For this review, take the finished solid that the model builds, in its own axes (mm). A direction names the side the tool comes from. Round coordinates to 2 decimals unless told otherwise and drop trailing zeros. Write each loop counter-clockwise with the first axis right and the second up, starting at its lowest first coordinate (ties: lowest second). Pieces come first, ordered by that corner, then holes. Notation, with made-up numbers: (0.25, 13.25) - (22.25, 13.25) arc R19 ccw to (22.25, 22.25) - close; hole circle Ø1 at (-1, 82). An arc over 180 degrees is marked (long way). One line per item, written item: value. Start each with the question number.
Q1. Add section D-D on y = 15.5. Write out the cut boundary in (x, z), and give its area (3 significant figures).
Q2. Mouldability with a two-part tool opening along X and no side actions: class faces 4 (the face through (22.805, 25.487, 0.74)), 5 (the face through (38, 24, 1)), 6 (the face through (0, -14, 1)), 7 (the face through (19, 32.5, 1)) as +X half, -X half, draft (parallel to the pull), parting line (faces both ways), or undercut.
Q3. Add section A-A on x = 33. Write out the cut boundary in (y, z).
Q4. Tool access review of faces 1 (the face through (18, 0, 1)), 2 (the face through (2.6, 20.92, 0.76)), 3 (the face through (1.141, 31.297, 0.76)): name each direction out of +Z, -Z, +X, -X, +Y, -Y from which nothing blocks a thin tool from reaching the whole face with its end or side.
Q5. Add section B-B on z = 0.5. Write out the cut boundary in (x, y).
Q6. Add section C-C on y = 24. Write out the cut boundary in (x, z).
Q7. For probe 1 along Y at (x, z) = (33, 0.5); probe 2 along Y at (x, z) = (22, 0.9); probe 3 along X at (y, z) = (-25, 0.5), list the stretches that pass through material, from the lowest coordinate up.
```python
from build123d import *

# Parameters (mm, degrees)
ESQUISSE1_R             = 2.5
ESQUISSE1_R_2           = 1.5
BOSS_EXTRU_1_DEPTH      = 1.5
CONG_1_R                = 4
ENL_V_MAT_EXTRU_1_DEPTH = 51.024993753


with BuildPart() as part:
    # Esquisse1 → Boss.-Extru.1 (new body)
    with BuildSketch(Plane.XY):
        Polygon((38, -20), (38, -32.5), (0, -32.5), (0, 32.5), (38, 32.5), (38, 20), (18, 20), (18, -20), align=None)
        with Locations((8, 25)):
            Circle(ESQUISSE1_R, mode=Mode.SUBTRACT)
        with Locations((23, 24)):
            Circle(ESQUISSE1_R_2, mode=Mode.SUBTRACT)
        with Locations(Location((33, 24, 0), (0, 0, 180))):
            Circle(ESQUISSE1_R_2, mode=Mode.SUBTRACT)
        with Locations((33, -24)):
            Circle(ESQUISSE1_R_2, mode=Mode.SUBTRACT)
        with Locations(Location((23, -24, 0), (0, 0, 180))):
            Circle(ESQUISSE1_R_2, mode=Mode.SUBTRACT)
        with Locations(Location((8, -25, 0), (0, 0, 180))):
            Circle(ESQUISSE1_R, mode=Mode.SUBTRACT)
    extrude(amount=BOSS_EXTRU_1_DEPTH)

    # Congé1
    cong_1_edges = [part.edges().sort_by_distance(p)[0] for p in [
        (38, -32.5, 0.75),
        (0, -32.5, 0.75),
        (0, 32.5, 0.75),
        (38, 32.5, 0.75),
    ]]
    fillet(cong_1_edges, radius=CONG_1_R)

    # Esquisse2 → Enlèv. mat.-Extru.1 (cut, through all)
    with BuildSketch(Plane.XY.offset(1.5)):
        Polygon((0, 21.617026009), (5.268332191, 20.205380653), (0, 0.543697246), align=None)
    extrude(amount=-ENL_V_MAT_EXTRU_1_DEPTH, mode=Mode.SUBTRACT)


solid = part.part
```
Result set:
1. outline: (4.01, 0) - (18, 0) - (18, 1.5) - (4.01, 1.5) - close
1. area: 21.0 mm^2
2. face 4: undercut
2. face 5: +X half
2. face 6: -X half
2. face 7: draft
3. outline: (-32.5, 0) - (-25.5, 0) - (-25.5, 1.5) - (-32.5, 1.5) - close; (-22.5, 0) - (-20, 0) - (-20, 1.5) - (-22.5, 1.5) - close; (20, 0) - (22.5, 0) - (22.5, 1.5) - (20, 1.5) - close; (25.5, 0) - (32.5, 0) - (32.5, 1.5) - (25.5, 1.5) - close
4. face 1: +Z, -Z, +X
4. face 2: +Z, -Z, -X
4. face 3: +Z, -Z, -X, +Y
5. outline: (0, -28.5) arc R4 ccw to (4, -32.5) - (34, -32.5) arc R4 ccw to (38, -28.5) - (38, -20) - (18, -20) - (18, 20) - (38, 20) - (38, 28.5) arc R4 ccw to (34, 32.5) - (4, 32.5) arc R4 ccw to (0, 28.5) - (0, 21.62) - (5.27, 20.21) - (0, 0.54) - close; hole circle Ø5 at (8, -25); hole circle Ø5 at (8, 25); hole circle Ø3 at (23, -24); hole circle Ø3 at (23, 24); hole circle Ø3 at (33, -24); hole circle Ø3 at (33, 24)
6. outline: (0, 0) - (5.71, 0) - (5.71, 1.5) - (0, 1.5) - close; (10.29, 0) - (21.5, 0) - (21.5, 1.5) - (10.29, 1.5) - close; (24.5, 0) - (31.5, 0) - (31.5, 1.5) - (24.5, 1.5) - close; (34.5, 0) - (38, 0) - (38, 1.5) - (34.5, 1.5) - close
7. probe 1: y = -32.5 to -25.5, -22.5 to -20, 20 to 22.5, 25.5 to 32.5
7. probe 2: y = -32.5 to -25.12, -22.88 to -20, 20 to 22.88, 25.12 to 32.5
7. probe 3: x = 0 to 5.5, 10.5 to 21.88, 24.12 to 31.88, 34.12 to 38
